CAD build for the part. Positions are in the model's coordinates, mm. Face numbers are marked on the shaded views. Give positions to 0.01 mm unless a question says otherwise; leave off trailing zeros. Loops run counter-clockwise (first coordinate to the right, second up) from the corner with the lowest first, then second, coordinate; pieces in that order, holes last.
Item 1: Saw through at A-A on y = -0.5. Give the cut face in (x, z).
Item 2: Probe probe 1 along X at (y, z) = (0, 0); probe 2 along Z at (x, y) = (0.7, 1); probe 3 along Y at (x, z) = (-0.2, -1.3). List the from-to ranges inside material, lowest first.
Item 3: Drop flat-ended pins along their axis: P1, Ø1.8, axis at x = 0, z = 0, coming from the +Y side; P2, Ø1.5, axis at x = -1, y = 1.5, coming from the +Z side; P3, Ø1.6, axis at x = 0, z = 0.5, coming from the -Y side. Give the stop position or say it passes through.
Item 4: Mould opens along Z. For the marked faces 1, 2 and 3 say: released by +Z, released by -Z, zero draft, split by the parting line, or undercut.
from build123d import *

# Parameters (mm, degrees)
SKETCH1_R           = 1.25
SKETCH1_R_2         = 1
BOSS_EXTRUDE1_DEPTH = 4
SKETCH2_R           = 1
BOSS_EXTRUDE2_DEPTH = 1.01


with BuildPart() as part:
    # Sketch1 → Boss-Extrude1 (new body)
    with BuildSketch(Plane(origin=(0, 0, 0), x_dir=(1, 0, 0), z_dir=(0, 1, 0))):
        with Locations(Location((0, 0, 0), (0, 0, 270))):
            Circle(SKETCH1_R)
        with Locations(Location((0, 0, 0), (0, 0, 270))):
            Circle(SKETCH1_R_2, mode=Mode.SUBTRACT)
    boss_extrude1 = extrude(amount=BOSS_EXTRUDE1_DEPTH)

    # Sketch2 → Boss-Extrude2 (add)
    with BuildSketch(Plane(origin=(0, 4, 0), x_dir=(1, 0, 0), z_dir=(0, 1, 0))):
        Polygon((-0.740860879, 1.418141445), (-0.881677878, 1.213525492), (-1.11979406, 1.142830374), (-1.253620181, 0.994201408), (-1.299038106, 0.75), (-1.487813767, 0.58856622), (-1.549617166, 0.398354916), (-1.491782843, 0.156792695), (-1.598576957, -0.067466381), (-1.577671264, -0.26637076), (-1.426584774, -0.463525492), (-1.432931669, -0.711833431), (-1.332931669, -0.885038512), (-1.114717238, -1.00369591), (-1.019519477, -1.233118014), (-0.857716078, -1.350675064), (-0.610104965, -1.370318186), (-0.429823106, -1.54118529), (-0.234193585, -1.582767628), (0, -1.5), (0.234193585, -1.582767628), (0.429823106, -1.54118529), (0.610104965, -1.370318186), (0.857716078, -1.350675064), (1.019519477, -1.233118014), (1.114717238, -1.00369591), (1.332931669, -0.885038512), (1.432931669, -0.711833431), (1.426584774, -0.463525492), (1.577671264, -0.26637076), (1.598576957, -0.067466381), (1.491782843, 0.156792695), (1.549617166, 0.398354916), (1.487813767, 0.58856622), (1.299038106, 0.75), (1.253620181, 0.994201408), (1.11979406, 1.142830374), (0.881677878, 1.213525492), (0.740860879, 1.418141445), (0.558151787, 1.499488774), (0.311867536, 1.467221401), (0.1, 1.596871942), (-0.1, 1.596871942), (-0.311867536, 1.467221401), (-0.558151787, 1.499488774), align=None)
        with Locations(Location((0, 0, 0), (0, 0, 270))):
            Circle(SKETCH2_R, mode=Mode.SUBTRACT)
    boss_extrude2 = extrude(amount=BOSS_EXTRUDE2_DEPTH)

    # Mirror1: Boss-Extrude1, Boss-Extrude2 across plane
    add(boss_extrude1.mirror(Plane.ZX))
    add(boss_extrude2.mirror(Plane.ZX))


solid = part.part
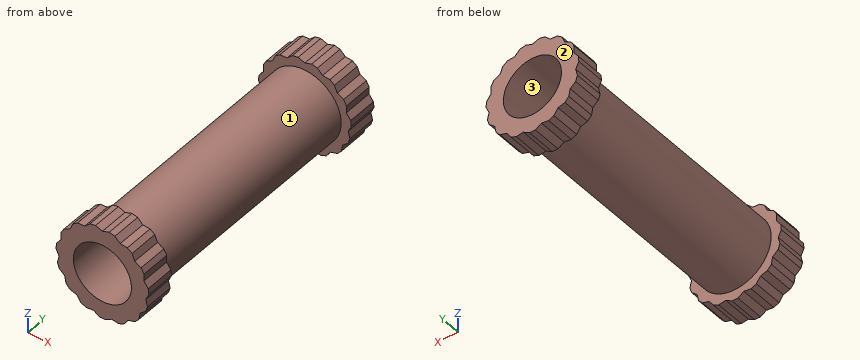
Results below:
1. outline: circle Ø2.5 at (0, 0); hole circle Ø2 at (0, 0)
2. probe 1: x = -1.25 to -1, 1 to 1.25
2. probe 2: z = -1.04 to -0.71, 0.71 to 1.04
2. probe 3: y = -5.01 to -4, 4 to 5.01
3. P1: passes through
3. P2: stops at z = 1.22
3. P3: stops at y = -5.01
4. face 1: split by the parting line
4. face 2: zero draft
4. face 3: undercut
